```python
from build123d import *

# Parameters (mm, degrees)
BOX007_W                  = 30
BOX007_H                  = 20
BOX007_DEPTH              = 10
BOX005_W                  = 12
BOX005_H                  = 60
BOX005_DEPTH              = 30
BOX006_W                  = 12
BOX006_H                  = 60
BOX006_DEPTH              = 30
BOX004_W                  = 50
BOX004_H                  = 30
BOX004_DEPTH              = 19
BOX004_PLACEMENT_ANGLE    = 15
CYLINDER012_R             = 5.1
CYLINDER012_DEPTH         = 50
CYLINDER007_R             = 7.5
CYLINDER007_DEPTH         = 70
CYLINDER009_R             = 6.5
CYLINDER009_DEPTH         = 70
CYLINDER010_R             = 7.5
CYLINDER010_DEPTH         = 70
CYLINDER011_R             = 6.5
CYLINDER011_DEPTH         = 70
FUSION007_PLACEMENT_ANGLE = 180
CYLINDER008_R             = 5.1
CYLINDER008_DEPTH         = 70
BOX003_W                  = 57
BOX003_H                  = 59
BOX003_DEPTH              = 20
CYLINDER004_R             = 6.35
CYLINDER004_DEPTH         = 50
BOX_W                     = 40
BOX_H                     = 20
BOX_DEPTH                 = 30
BOX_PLACEMENT_ANGLE       = 15
CYLINDER001_R             = 5
CYLINDER001_DEPTH         = 50
CYLINDER006_R             = 6.35
CYLINDER006_DEPTH         = 50
BOX001_W                  = 40
BOX001_H                  = 20
BOX001_DEPTH              = 30
BOX001_PLACEMENT_ANGLE    = 15
CYLINDER005_R             = 5
CYLINDER005_DEPTH         = 50
FUSION003_PLACEMENT_ANGLE = 180
BOX002_W                  = 24
BOX002_H                  = 39
BOX002_DEPTH              = 10


with BuildPart() as cube007:
    # Box007 → Box007 (new body)
    with BuildSketch(Plane(origin=(-16, 20, 42), x_dir=(1, 0, 0), z_dir=(0, 0, 1))):
        with Locations((15, 10)):
            Rectangle(BOX007_W, BOX007_H)
    extrude(amount=BOX007_DEPTH)


with BuildPart() as cone:
    # Cone → Cone (revolve)
    with BuildSketch(Plane(origin=(0, 13, 52), x_dir=(-1, 0, 0), z_dir=(0, -1, 0))):
        Polygon((0, 0), (5, 0), (6, 10), (0, 10), align=None)
    revolve(axis=Axis((0, 13, 52), (0, 0, -1)))


with BuildPart() as cube005:
    # Box005 → Box005 (new body)
    with BuildSketch(Plane(origin=(14, -29, 23), x_dir=(1, 0, 0), z_dir=(0, 0, 1))):
        with Locations((6, 30)):
            Rectangle(BOX005_W, BOX005_H)
    extrude(amount=BOX005_DEPTH)


with BuildPart() as fusion009:
    # Box006 → Box006 (new body)
    with BuildSketch(Plane(origin=(-26, -29, 23), x_dir=(1, 0, 0), z_dir=(0, 0, 1))):
        with Locations((6, 30)):
            Rectangle(BOX006_W, BOX006_H)
    extrude(amount=BOX006_DEPTH)

    # Fusion009: union Cube005
    add(cube005.part)


with BuildPart() as cube004:
    # Box004 → Box004 (new body)
    with BuildSketch(Plane.XY):
        with Locations((25, 15)):
            Rectangle(BOX004_W, BOX004_H)
    extrude(amount=BOX004_DEPTH)


with BuildPart() as cube004_1:
    # Box004 placement: moved
    add(cube004.part.moved(Location((-24, 7.965926, 22.258819))).rotate(Axis((-24, 7.965926, 22.258819), (1, 0, 0)), BOX004_PLACEMENT_ANGLE))


with BuildPart() as obj1:
    # Cylinder012 → Cylinder012 (new body)
    with BuildSketch(Plane(origin=(0, -12.5, -17), x_dir=(1, 0, 0), z_dir=(0, 0, 1))):
        Circle(CYLINDER012_R)
    extrude(amount=CYLINDER012_DEPTH)


with BuildPart() as obj2:
    # Cylinder007 → Cylinder007 (new body)
    with BuildSketch(Plane.XY):
        Circle(CYLINDER007_R)
    extrude(amount=CYLINDER007_DEPTH)


with BuildPart() as fusion006:
    # Cylinder009 → Cylinder009 (new body)
    with BuildSketch(Plane(origin=(0, 6.5, 0), x_dir=(1, 0, 0), z_dir=(0, 0, 1))):
        Circle(CYLINDER009_R)
    extrude(amount=CYLINDER009_DEPTH)

    # Fusion006: union obj2
    add(obj2.part)


with BuildPart() as obj3:
    # Cylinder010 → Cylinder010 (new body)
    with BuildSketch(Plane.XY):
        Circle(CYLINDER010_R)
    extrude(amount=CYLINDER010_DEPTH)


with BuildPart() as fusion008:
    # Cylinder011 → Cylinder011 (new body)
    with BuildSketch(Plane(origin=(0, 6.5, 0), x_dir=(1, 0, 0), z_dir=(0, 0, 1))):
        Circle(CYLINDER011_R)
    extrude(amount=CYLINDER011_DEPTH)

    # Fusion007: union obj3
    add(obj3.part)


with BuildPart() as fusion008_1:
    # Fusion007 placement: moved
    add(fusion008.part.rotate(Axis((0, 0, 0), (0, 0, 1)), FUSION007_PLACEMENT_ANGLE))

    # Fusion008: union Fusion006
    add(fusion006.part)


with BuildPart() as cylinder008:
    # Cylinder008 → Cylinder008 (new body)
    with BuildSketch(Plane(origin=(0, 12.5, 0), x_dir=(1, 0, 0), z_dir=(0, 0, 1))):
        Circle(CYLINDER008_R)
    extrude(amount=CYLINDER008_DEPTH)


with BuildPart() as cube003:
    # Box003 → Box003 (new body)
    with BuildSketch(Plane(origin=(-29.5, -29, 51.5), x_dir=(1, 0, 0), z_dir=(0, 0, 1))):
        with Locations((28.5, 29.5)):
            Rectangle(BOX003_W, BOX003_H)
    extrude(amount=BOX003_DEPTH)


with BuildPart() as obj4:
    # Cylinder004 → Cylinder004 (new body)
    with BuildSketch(Plane.XY):
        Circle(CYLINDER004_R)
    extrude(amount=CYLINDER004_DEPTH)


with BuildPart() as cube:
    # Box → Box (new body)
    with BuildSketch(Plane.XY):
        with Locations((20, 10)):
            Rectangle(BOX_W, BOX_H)
    extrude(amount=BOX_DEPTH)


with BuildPart() as cube_1:
    # Box placement: moved
    add(cube.part.moved(Location((-19.558238, 7, 39.759763))).rotate(Axis((-19.558238, 7, 39.759763), (0, 1, 0)), BOX_PLACEMENT_ANGLE))


with BuildPart() as fusion001:
    # Cylinder001 → Cylinder001 (new body)
    with BuildSketch(Plane(origin=(0, 12.5, 0), x_dir=(1, 0, 0), z_dir=(0, 0, 1))):
        Circle(CYLINDER001_R)
    extrude(amount=CYLINDER001_DEPTH)

    # Fusion: union Cube
    add(cube_1.part)

    # Fusion001: union obj4
    add(obj4.part)


with BuildPart() as obj5:
    # Cylinder006 → Cylinder006 (new body)
    with BuildSketch(Plane.XY):
        Circle(CYLINDER006_R)
    extrude(amount=CYLINDER006_DEPTH)


with BuildPart() as cube001:
    # Box001 → Box001 (new body)
    with BuildSketch(Plane.XY):
        with Locations((20, 10)):
            Rectangle(BOX001_W, BOX001_H)
    extrude(amount=BOX001_DEPTH)


with BuildPart() as cube001_1:
    # Box001 placement: moved
    add(cube001.part.moved(Location((-19.558238, 7, 39.759763))).rotate(Axis((-19.558238, 7, 39.759763), (0, 1, 0)), BOX001_PLACEMENT_ANGLE))


with BuildPart() as fusion004:
    # Cylinder005 → Cylinder005 (new body)
    with BuildSketch(Plane(origin=(0, 12.5, 0), x_dir=(1, 0, 0), z_dir=(0, 0, 1))):
        Circle(CYLINDER005_R)
    extrude(amount=CYLINDER005_DEPTH)

    # Fusion002: union Cube001
    add(cube001_1.part)

    # Fusion003: union obj5
    add(obj5.part)


with BuildPart() as fusion004_1:
    # Fusion003 placement: moved
    add(fusion004.part.rotate(Axis((0, 0, 0), (0, 0, 1)), FUSION003_PLACEMENT_ANGLE))

    # Fusion004: union Fusion001
    add(fusion001.part)


with BuildPart() as cut007:
    # Box002 → Box002 (new body)
    with BuildSketch(Plane(origin=(-12, -13, 41.5), x_dir=(1, 0, 0), z_dir=(0, 0, 1))):
        with Locations((12, 19.5)):
            Rectangle(BOX002_W, BOX002_H)
    extrude(amount=BOX002_DEPTH)

    # Fusion005: union Fusion004
    add(fusion004_1.part)

    # Cut: cut Cube003
    add(cube003.part, mode=Mode.SUBTRACT)

    # Cut001: cut Cylinder008
    add(cylinder008.part, mode=Mode.SUBTRACT)

    # Cut002: cut Fusion008
    add(fusion008_1.part, mode=Mode.SUBTRACT)

    # Cut003: cut obj1
    add(obj1.part, mode=Mode.SUBTRACT)

    # Cut004: cut Cube004
    add(cube004_1.part, mode=Mode.SUBTRACT)

    # Cut005: cut Fusion009
    add(fusion009.part, mode=Mode.SUBTRACT)

    # Cut006: cut Cone
    add(cone.part, mode=Mode.SUBTRACT)

    # Cut007: cut Cube007
    add(cube007.part, mode=Mode.SUBTRACT)


solid = cut007.part
```
Here's how the part is built. I have some questions about the finished solid (model axes, mm). A direction names the side the tool comes from. Round coordinates to 2 decimals unless told otherwise and drop trailing zeros. Write each loop counter-clockwise with the first axis right and the second up, starting at its lowest first coordinate (ties: lowest second). Pieces come first, ordered by that corner, then holes. Notation, with made-up numbers: M -25.75,45.5 L 30.25,45.5 A17 ccw 30.25,66.5 Z; hole C -10.75,-20 d9. An arc over 180 degrees is marked long. Answer as CSV lines item,"result". Start each with the question number.
1. Thinking about a two-plate mould opening in X: for faces 6 (the conical face through (-0.15, 18.4, 47.96)), 7 (the flat face through (-14, -17, 41)), 8 (the cylindrical face through (7.5, -0.1, 46.4)), 9 (the flat face through (-6.4, -8.4, 51.5)), which applies, released by +X, released by -X, zero draft, split by the parting line, or undercut?
2. I need wall thicknesses on probe 1 along X at (y, z) = (-6.5, 46.75); probe 2 along Y at (x, z) = (0, 45.5); probe 3 along Y at (x, z) = (0.5, 48.75). Which ranges of each line are inside material? Lowest first, please.
3. Suppose I cut it at A-A on y = -6.5. Write out the boundary of the cut face in (x, z).
4. Suppose I cut it at C-C on x = 0. Write out the boundary of the cut face in (y, z).
5. I'm going to push flat-ended pins straight in: pin 1 Ø2 at (y, z) = (12, 40) entering from +X; pin 2 Ø8 at (y, z) = (0, 48.5) entering from +X; pin 3 Ø3.5 at (x, y) = (1, -13) entering from -Z; pin 4 Ø8.5 at (x, z) = (-10.5, 42) entering from +Y. Where does each tip first touch, or does it pass through?
6. On a 3-axis mill with a long thin cutter (end or side, diameter ignored), from which of +Z, -Z, +X, -X, +Y, -Y can I reach the whole of each face in a straight line? I mean faces 1 (the flat face through (10, 0, 41.5)), 2 (the flat face through (-11, -7, 39)), 3 (the flat face through (13, 7, 47)), 4 (the cylindrical face through (-7.5, 0.1, 46.4)), 5 (the flat face through (11, -7, 41)). Say none if no direction works.
7. Suppose I cut it at B-B on z = 50. Write out the boundary of the cut face in (x, y), then the cut area to 3 significant figures.
8. Suppose I cut it at D-D on y = -12.5. Write out the boundary of the cut face in (x, z).
Check result:
1,face 6,"undercut"
1,face 7,"released by -X"
1,face 8,"undercut"
1,face 9,"zero draft"
2,probe 1,"x = -12 to -6.5, 6.5 to 12"
2,probe 2,"y = -27 to -13, 18.65 to 20"
2,probe 3,"y = -27 to -12.98, 18.3 to 20"
3,outline,"M -12,41.5 L -6.5,41.5 L -6.5,51.5 L -12,51.5 Z; M 6.5,41.5 L 12,41.5 L 12,51.5 L 6.5,51.5 Z"
4,outline,"M -27,34.52 L -17.5,34.52 L -17.5,33 L -13,33 L -13,51.5 L -27,51.5 Z; M 18.05,51.5 L 18.72,44.81 L 20,45.15 L 20,51.5 Z"
5,pin 1,"passes through"
5,pin 2,"stops at x = 12"
5,pin 3,"stops at z = 33"
5,pin 4,"stops at y = 20"
6,face 1,"-Z, +X, -X, +Y"
6,face 2,"-Z, -X"
6,face 3,"+Z, -Z, +X"
6,face 4,"+Z, -Z"
6,face 5,"-Z, +X"
7,outline,"M -14,-27 L 14,-27 L 14,-7 L 12,-7 L 12,7 L 14,7 L 14,20 L -14,20 L -14,7 L -12,7 L -12,-7 L -14,-7 Z; hole M -6.13,-4.33 A6.5 ccw long 6.13,-4.33 A7.5 ccw 6.13,4.33 A6.5 ccw 4.83,10.85 A5.1 ccw 5.04,11.72 A5.2 ccw long -5.04,11.72 A5.1 ccw -4.83,10.85 A6.5 ccw -6.13,4.33 A7.5 ccw Z"
7,area,"900 mm2"
8,outline,"M -14,30.77 L -5,33.18 L -5,33 L -2.5,33 L -2.5,51.5 L -14,51.5 Z; M 2.5,33 L 5,33 L 5,35.86 L 14,38.27 L 14,51.5 L 2.5,51.5 Z"
